Work out the finished part from the listing and answer in its coordinate system (mm). A direction names the side the tool comes from. Round coordinates to 2 decimals unless told otherwise and drop trailing zeros. Loops run counter-clockwise (first coordinate to the right, second up) from the corner with the lowest first, then second, coordinate; pieces in that order, holes last. Notation, with made-up numbers: M -16,-7 L 5,-7 A30 cw 5,15 Z; hole C 48,55 d9. An arc over 180 degrees is marked long. One line per item, written item: value.
```python
from build123d import *

# Parameters (mm, degrees)
SKETCH1_W           = 250
SKETCH1_H           = 175
BOSS_EXTRUDE1_DEPTH = 30
FILLET1_R           = 5
SKETCH3_W           = 240
SKETCH3_H           = 165
CUT_EXTRUDE1_DEPTH  = 25
SKETCH4_R           = 2.5
SKETCH4_R_2         = 1.25
BOSS_EXTRUDE2_DEPTH = 10


with BuildPart() as part:
    # Sketch1 → Boss-Extrude1 (new body)
    with BuildSketch(Plane(origin=(0, 0, 0), x_dir=(1, 0, 0), z_dir=(0, 1, 0))):
        Rectangle(SKETCH1_W, SKETCH1_H)
    extrude(amount=BOSS_EXTRUDE1_DEPTH)

    # Fillet1
    fillet1_edges = [part.edges().sort_by_distance(p)[0] for p in [
        (125, 15, 87.5),
        (-125, 15, 87.5),
        (-125, 15, -87.5),
        (125, 15, -87.5),
    ]]
    fillet(fillet1_edges, radius=FILLET1_R)

    # Sketch3 → Cut-Extrude1 (cut)
    with BuildSketch(Plane(origin=(0, 30, 0), x_dir=(1, 0, 0), z_dir=(0, 1, 0))):
        Rectangle(SKETCH3_W, SKETCH3_H)
    extrude(amount=-CUT_EXTRUDE1_DEPTH, mode=Mode.SUBTRACT)

    # Sketch4 → Boss-Extrude2 (add)
    # profile 1 of 4: a face of its own
    with BuildSketch(Plane(origin=(0, 5, 0), x_dir=(1, 0, 0), z_dir=(0, 1, 0))):
        with Locations(Location((-105.355, 71.49, 0), (0, 0, 270))):
            Circle(SKETCH4_R)
        with Locations(Location((-105.355, 71.49, 0), (0, 0, 270))):
            Circle(SKETCH4_R_2, mode=Mode.SUBTRACT)
    # profile 2 of 4: a face of its own
    with BuildSketch(Plane(origin=(0, 5, 0), x_dir=(1, 0, 0), z_dir=(0, 1, 0))):
        with Locations(Location((105.355, 71.49, 0), (0, 0, 270))):
            Circle(SKETCH4_R)
        with Locations(Location((105.355, 71.49, 0), (0, 0, 270))):
            Circle(SKETCH4_R_2, mode=Mode.SUBTRACT)
    # profile 3 of 4: a face of its own
    with BuildSketch(Plane(origin=(0, 5, 0), x_dir=(1, 0, 0), z_dir=(0, 1, 0))):
        with Locations(Location((105.355, -71.49, 0), (0, 0, 270))):
            Circle(SKETCH4_R)
        with Locations(Location((105.355, -71.49, 0), (0, 0, 270))):
            Circle(SKETCH4_R_2, mode=Mode.SUBTRACT)
    # profile 4 of 4: a face of its own
    with BuildSketch(Plane(origin=(0, 5, 0), x_dir=(1, 0, 0), z_dir=(0, 1, 0))):
        with Locations(Location((-105.355, -71.49, 0), (0, 0, 270))):
            Circle(SKETCH4_R)
        with Locations(Location((-105.355, -71.49, 0), (0, 0, 270))):
            Circle(SKETCH4_R_2, mode=Mode.SUBTRACT)
    extrude(amount=BOSS_EXTRUDE2_DEPTH)


solid = part.part
```
1) Find section B-B (x = 18.5). Give the vertices of the cut face in (y, z), then the cut area to 4 significant figures.
Check values:
outline: M 0,-87.5 L 30,-87.5 L 30,-82.5 L 5,-82.5 L 5,82.5 L 30,82.5 L 30,87.5 L 0,87.5 Z
area: 1,125 mm2
2) Find section A-A (y = 21.75). Give the vertices of the cut face in (x, z).
Check values:
outline: M -125,-82.5 A5 ccw -120,-87.5 L 120,-87.5 A5 ccw 125,-82.5 L 125,82.5 A5 ccw 120,87.5 L -120,87.5 A5 ccw -125,82.5 Z; hole M -120,-82.5 L 120,-82.5 L 120,82.5 L -120,82.5 Z
3) Each of these flat-tipped pins is pushed along its axis until it touches: pin 1 (0.8 mm diameter, centred on x = -105.5, z = 71.5, fed in from +Y); pin 2 (2 mm diameter, centred on x = -38, z = 9, fed in from -Y); pin 3 (2.5 mm diameter, centred on x = 104.5, z = -72, fed in from +Y). Where does it stop, or does it pass through?
Check values:
pin 1: y = 5
pin 2: y = 0
pin 3: y = 15
4) Find the intervals of material crossed by probe 1 along X at (y, z) = (8, 71.49) (3 decimals); probe 2 along Z at (x, y) = (71.5, 17); probe 3 along X at (y, z) = (12.5, 3), in increasing order. Write a range as from..to.
Check values:
probe 1: -125..-120, -107.855..-106.605, -104.105..-102.855, 102.855..104.105, 106.605..107.855, 120..125
probe 2: -87.5..-82.5, 82.5..87.5
probe 3: -125..-120, 120..125
5) The mould has two halves that part along X. Classify faces 3 (the face through (-120, 18, 1)), 4 (the face through (-125, 15, 1)), 5 (the face through (-2, 15, -87.5)), 6 (the face through (107, 15, -71)): +X half, -X half, draft (parallel to the pull), parting line (faces both ways), or undercut.
Check values:
face 3: undercut
face 4: -X half
face 5: draft
face 6: undercut
6) Find section C-C (z = -60.5). Give the vertices of the cut face in (x, y).
Check values:
outline: M -125,0 L 125,0 L 125,30 L 120,30 L 120,5 L -120,5 L -120,30 L -125,30 Z
7) For faces 1 (the face through (105, 15, 70)), 2 (the face through (123.5, 15.21, 86.07)), determine the directions among +Z, -Z, +X, -X, +Y, -Y from which every point of the face is accessible in a straight line to the end or side of a thin tool.
Check values:
face 1: +Y
face 2: +Z, +X, +Y, -Y
